The listing builds one solid part. Answer for the finished solid, in the listing's coordinates (mm). Face numbers are marked on the shaded views. A direction names the side the tool comes from. Coordinates: 2 decimals unless noted, no trailing zeros. Order: outer loops, then holes, each group sorted by start corner. A loop starts at its lowest first (then second) coordinate and runs counter-clockwise, first axis right, second up. Notation, with made-up numbers: (56.5, 45.25) -> (73.5, 45.25) arc R10 cw to (73.5, 63.25) -> close; hole circle Ø3 at (45, 20.5). An arc over 180 degrees is marked (long way). Write item = value, one per line. Start each with the question number.
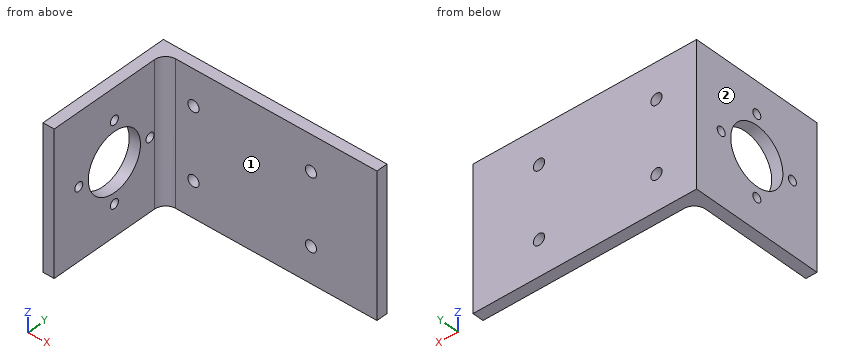
```python
from build123d import *

# Parameters (mm, degrees)
BOSS_EXTRUDE1_DEPTH = 63.5
SKETCH2_R           = 13
SKETCH2_R_2         = 2
CUT_EXTRUDE1_DEPTH  = 5
SKETCH4_R           = 2.5
CUT_EXTRUDE3_DEPTH  = 10


with BuildPart() as part:
    # Sketch1 → Boss-Extrude1 (new body)
    with BuildSketch(Plane.XY):
        with BuildLine():
            Line((0, 0), (0, 60))
            Line((0, 60), (100, 60))
            Line((100, 60), (100, 55))
            Line((100, 55), (10, 55))
            ThreePointArc((10, 55), (6.464466094, 53.535533906), (5, 50))
            Line((5, 50), (5, 0))
            Line((5, 0), (0, 0))
        make_face()
    extrude(amount=BOSS_EXTRUDE1_DEPTH)

    # Sketch2 → Cut-Extrude1 (cut)
    with BuildSketch(Plane.ZY):
        with Locations((31.75, 30)):
            Circle(SKETCH2_R)
        with Locations((49.5, 30)):
            Circle(SKETCH2_R_2)
        with Locations((31.75, 12.25)):
            Circle(SKETCH2_R_2)
        with Locations((14, 30)):
            Circle(SKETCH2_R_2)
        with Locations((31.75, 47.75)):
            Circle(SKETCH2_R_2)
    extrude(amount=-CUT_EXTRUDE1_DEPTH, mode=Mode.SUBTRACT)

    # Sketch4 → Cut-Extrude3 (cut)
    with BuildSketch(Plane(origin=(0, 60, 0), x_dir=(1, 0, 0), z_dir=(0, 1, 0))):
        with Locations((70.47984065, -47.625)):
            Circle(SKETCH4_R)
        with Locations((17.94984065, -47.625)):
            Circle(SKETCH4_R)
        with Locations((17.94984065, -15.875)):
            Circle(SKETCH4_R)
        with Locations((70.47984065, -15.875)):
            Circle(SKETCH4_R)
    extrude(amount=-CUT_EXTRUDE3_DEPTH, mode=Mode.SUBTRACT)


solid = part.part
```
Item 1: Section D-D, the plane x = 60.5 is taken. Give the vertices of the cut face in (y, z), then the cut area to 4 significant figures.
Item 2: Which of the six approach directions +Z, -Z, +X, -X, +Y, -Y give full straight-line access (tool end or side, diameter ignored) to the marked faces 1 and 2?
Item 3: Each of these flat-tipped pins is pushed along its axis until it touches: pin 1 (3 mm diameter, centred on x = 89.5, z = 40, fed in from -Y); pin 2 (3 mm diameter, centred on y = 36, z = 6.5, fed in from +X); pin 3 (4 mm diameter, centred on x = 17.95, z = 15.88, fed in from -Y). Where does it stop, or does it pass through?
Item 4: Section C-C, the plane z = 5 is taken. Give the vertices of the cut face in (x, y), then the cut area to 3 significant figures.
Item 5: Section B-B, the plane y = 47.75 is taken. Give the vertices of the cut face in (x, z), then the cut area to 4 significant figures.
Item 6: Section A-A, the plane z = 31.75 is taken. Give the vertices of the cut face in (x, y), then the cut area to 3 significant figures.
Item 7: Consider probe 1 along Y at (x, z) = (1.2, 31.75); probe 2 along Y at (x, z) = (2.55, 49.5); probe 3 along X at (y, z) = (29.5, 7). Determine where each line is inside the solid, lowest interval first.
A:
q1.outline = (55, 0) -> (60, 0) -> (60, 63.5) -> (55, 63.5) -> close
q1.area = 317.5 mm^2
q2.face_1 = +Z, -Z, +X, -Y
q2.face_2 = +Z, -Z, -X, +Y, -Y
q3.pin_1 = 55
q3.pin_2 = 5
q3.pin_3 = through
q4.outline = (0, 0) -> (5, 0) -> (5, 50) arc R5 cw to (10, 55) -> (100, 55) -> (100, 60) -> (0, 60) -> close
q4.area = 780 mm^2
q5.outline = (0, 0) -> (5, 0) -> (5, 29.75) -> (0, 29.75) -> close; (0, 33.75) -> (5, 33.75) -> (5, 63.5) -> (0, 63.5) -> close
q5.area = 297.5 mm^2
q6.outline = (0, 0) -> (5, 0) -> (5, 10.25) -> (0, 10.25) -> close; (0, 14.25) -> (5, 14.25) -> (5, 17) -> (0, 17) -> close; (0, 43) -> (5, 43) -> (5, 45.75) -> (0, 45.75) -> close; (0, 49.75) -> (5, 49.75) -> (5, 50) arc R5 cw to (10, 55) -> (100, 55) -> (100, 60) -> (0, 60) -> close
q6.area = 610 mm^2
q7.probe_1 = 0 to 10.25, 14.25 to 17, 43 to 45.75, 49.75 to 60
q7.probe_2 = 0 to 28, 32 to 60
q7.probe_3 = 0 to 5
